Geometry: final body of the model. Coordinates: model frame, mm. Face numbers are marked on the shaded views. Round coordinates to 2 decimals unless told otherwise and drop trailing zeros. Loops run counter-clockwise (first coordinate to the right, second up) from the corner with the lowest first, then second, coordinate; pieces in that order, holes last. Notation, with made-up numbers: M 13.25,-10.5 L 42.25,-10.5 A14 ccw 42.25,13.5 Z; hole C 75.5,86 d3. An arc over 180 degrees is marked long. Write each question's results on one line, items separated by ' | '.
```python
from build123d import *

# Parameters (mm, degrees)
F0_W     = 28.243152
F0_H     = 17.298024
F1_DEPTH = 5
F2_R     = 2
F3_R     = 3.167905
F4_DEPTH = 25


with BuildPart() as f1:
    # F0 (on Front) → F1 (new body)
    with BuildSketch(Plane.XZ):
        with Locations((14.121576, -8.649012)):
            Rectangle(F0_W, F0_H)
    extrude(amount=F1_DEPTH)

    # F2
    f2_edges = [f1.edges().sort_by_distance(p)[0] for p in [
        (14.121576, -5, -17.298024),
        (28.243152, -5, -8.649012),
        (14.121576, -5, 0),
        (0, -5, -8.649012),
    ]]
    fillet(f2_edges, radius=F2_R)

    # F3 (on face) → F4 (cut)
    with BuildSketch(Plane.XZ.offset(5)):
        with Locations((7.708723, -8.649012)):
            Circle(F3_R)
    extrude(amount=-F4_DEPTH, mode=Mode.SUBTRACT)


solid = f1.part
```
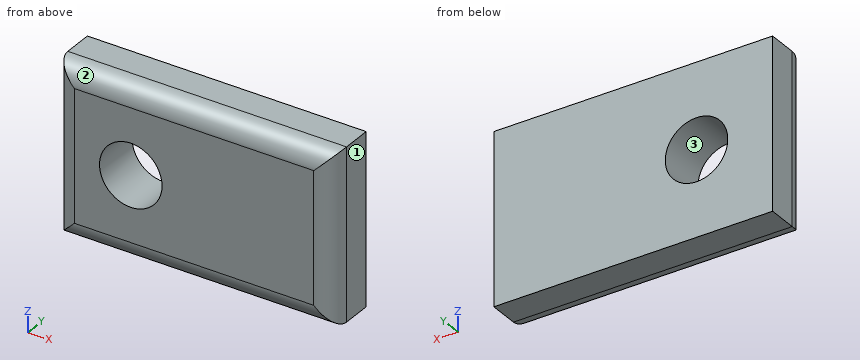
1. Section D-D (x = 3.5). Output: boundary loops of the cut face in (y, z).
Answer key:
outline: M -5,-15.3 A2 ccw -3,-17.3 L 0,-17.3 L 0,0 L -3,0 A2 ccw -5,-2 Z
2. Ray query, probe 1 along Z at (x, y) = (7.5, -4.4); probe 2 along X at (y, z) = (-0.85, -9.25); probe 3 along X at (y, z) = (-3.9, -12.5). Return the intervals inside material, ascending.
Answer key:
probe 1: z = -16.73 to -11.81, -5.49 to -0.57 | probe 2: x = 0 to 4.6, 10.82 to 28.24 | probe 3: x = 0.21 to 28.03
3. Section A-A (z = -10.5). Output: boundary loops of the cut face in (x, y), then the cut area to 3 significant figures.
Answer key:
outline: M 0,-3 A2 ccw 2,-5 L 5.14,-5 L 5.14,0 L 0,0 Z; M 10.28,-5 L 26.24,-5 A2 ccw 28.24,-3 L 28.24,0 L 10.28,0 Z | area: 114 mm²
4. Draft query along X for the marked faces 1, 2 and 3. Return one class per face: pulls with the +X half, pulls with the -X half, needs draft (parallel to the pull), parting line crosses it, or undercut.
Answer key:
face 1: pulls with the +X half | face 2: needs draft | face 3: undercut
5. Pin query (flat end, axial travel): P1, Ø10, axis at x = 11, z = -11.5, coming from the +Y side; P2, Ø5.5, axis at x = 7.71, z = -8.65, coming from the +Y side. Return the tip coordinate at first contact, or that it passes through.
Answer key:
P1: stops at y = 0 | P2: passes through
6. Section C-C (y = -1.1). Output: boundary loops of the cut face in (x, z), then the cut area to 3 significant figures.
Answer key:
outline: M 0,-17.3 L 28.24,-17.3 L 28.24,0 L 0,0 Z; hole C 7.71,-8.65 d6.34 | area: 457 mm²
7. Section B-B (x = 7.5). Output: boundary loops of the cut face in (y, z).
Answer key:
outline: M -5,-15.3 A2 ccw -3,-17.3 L 0,-17.3 L 0,-11.81 L -5,-11.81 Z; M -5,-5.49 L 0,-5.49 L 0,0 L -3,0 A2 ccw -5,-2 Z
